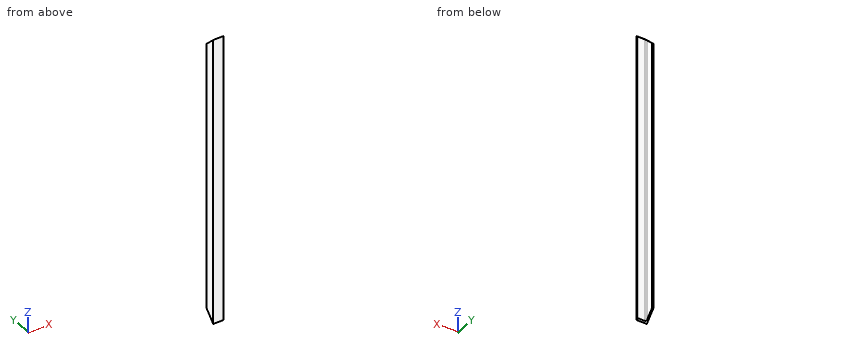
Autodesk Inventor part; units mm, degrees
ref_plane "Start plane" through (0, 0, 0) normal (0, 0, 1) x (1, 0, 0)
ref_plane "End plane" through (0, 0, 1092.2) normal (0, 0, 1) x (1, 0, 0)
ref_plane "Work Plane4" through (19.05, 0, 0) normal (0, 0.7071, -0.7071) x (1, 0, 0)
ref_plane "Start plane" through (0, 0, 0) normal (0, 0, 1) x (1, 0, 0)
ref_plane "End plane" through (0, 0, 1092.2) normal (0, 0, 1) x (1, 0, 0)
sketch "Sketch" plane through (0, 0, 0) normal (0, 0, 1) x (1, 0, 0)
  line L0 (38.1, 0) -> (0, 0)
  line L1 (0, 0) -> (0, 38.1)
  line L2 (0, 38.1) -> (2.4765, 38.1)
  line L3 (4.7625, 35.814) -> (4.7625, 9.5885)
  line L4 (9.5885, 4.7625) -> (35.814, 4.7625)
  line L5 (38.1, 2.4765) -> (38.1, 0)
  line L6 (0, -11.0414) -> (0, 31.5385) construction
  line L7 (-11.0414, 0) -> (31.5385, 0) construction
  arc A0 (4.7625, 9.5885) -> (9.5885, 4.7625) centre (9.5885, 9.5885) ccw
  arc A1 (4.7625, 35.814) -> (2.4765, 38.1) centre (2.4765, 35.814) ccw
  arc A2 (38.1, 2.4765) -> (35.814, 4.7625) centre (35.814, 2.4765) ccw
  line L8 (0, 48.4964) -> (0, -20.9644) construction
  line L9 (-20.9644, 0) -> (48.4964, 0) construction
  point P0 (4.7625, 38.1)
  point P1 (4.7625, 4.7625)
  point P2 (38.1, 4.7625)
  dimension "d0" = 38.1
  dimension "d1" = 38.1
  dimension "d2" = 4.7625
  dimension "d3" = 4.7625
  dimension "d10" = 0
  dimension "d11" = 0
  dimension "d14" = 4.826
  dimension "d15" = 2.286
extrude "Body" add sketch "Sketch" along normal up to surface (1092.2 mm away) from surface at 0
sketch "Sketch3" plane through (0, 0, 0) normal (0, 0, 1) x (1, 0, 0)
  line L0 (0, 0) -> (10, 0)
ref_plane "Work Plane3" through (0, 0, 0) normal (0, -1, 0) x (1, 0, 0)
sketch "Sketch4" plane through (0, 0, 0) normal (0, -1, 0) x (1, 0, 0)
  line L0 (-2, 0) -> (12, 0)
  line L1 (-2, 1092.2) -> (12, 1092.2)
  dimension "d17" = 1092.2
ref_plane "Work Plane4" through (19.05, 0, 0) normal (0, 0.7071, -0.7071) x (1, 0, 0)
split "Split1" plane through (19.05, 0, 0) removes the side toward (0, 0.7071, -0.7071)
ref_plane "Work Plane5" through (19.05, 0, 1092.2) normal (0, 0.7071, 0.7071) x (1, 0, 0)
split "Split2" plane through (19.05, 0, 1092.2) removes the side toward (0, 0.7071, 0.7071)
equation "\"d0\" = G_H"
equation "\"d1\" = G_H"
equation "\"d2\" = G_T"
equation "\"d3\" = G_T"
equation "\"d14\" = G_IR"
equation "\"d15\" = G_ER"
equation "\"d4\" = G_L"
equation "\"G_H\" = 38.1"
equation "\"G_T\" = 4.7625"
equation "\"G_ER\" = 2.286"
equation "\"G_IR\" = 4.826"
equation "\"G_L\" = d17"
equation "\"ex\" = 0"
equation "\"G_OFFSET_START\" = 0"
equation "\"G_OFFSET_END\" = 0"
equation "\"d13\" = G_OFFSET_END + B_L"
equation "\"B_L\" = 1092.2"
properties part number "AISC - L 1.5 x 1.5 x 3/16 - 43" material "Aluminum 6061"
The listing builds one solid part. Answer for the finished solid, in the listing's coordinates (mm). Give positions to 0.01 mm unless a question says otherwise; leave off trailing zeros. Order: outer loops, then holes, each group sorted by start corner. A loop starts at its lowest first (then second) coordinate and runs counter-clockwise, first axis right, second up. Notation, with made-up numbers: (-8.5, 14) - (22.5, 14) arc R22 ccw to (22.5, 41) - close; hole circle Ø5 at (-19.5, -13.5). An arc over 180 degrees is marked (long way). Use one line per item in the form item = value. Start each with the question number.
(1) Flat-ended cylindrical pins translate along their axes: pin 1 Ø8 at (y, z) = (14, 216) entering from +X; pin 2 Ø4 at (x, y) = (23, 4) entering from +Z; pin 3 Ø10 at (y, z) = (11.5, 571.5) entering from +X. Find the tip coordinate at first contact, or state that the pin passes through.
(2) Consider line 1 (X direction, y = 22, z = 981.5); line 2 (Y direction, x = 8.5, z = 665). Determine where each line is inside the solid, lowest interval first. Write a range as from..to.
(3) A cutting plane is placed at B-B, the plane x = 28.5. Write down the section's boundary in (y, z).
(4) A cutting plane is placed at C-C, the plane y = 17. Write down the section's boundary in (x, z), then the cut area to 3 significant figures.
(5) A cutting plane is placed at A-A, the plane z = 582. Write down the section's boundary in (x, y).
Ans:
q1.pin_1 = 4.76
q1.pin_2 = 1090.2
q1.pin_3 = 5.88
q2.line_1 = 0..4.76
q2.line_2 = 0..4.89
q3.outline = (0, 0) - (4.76, 4.76) - (4.76, 1087.44) - (0, 1092.2) - close
q4.outline = (0, 17) - (4.76, 17) - (4.76, 1075.2) - (0, 1075.2) - close
q4.area = 5,040 mm^2
q5.outline = (0, 0) - (38.1, 0) - (38.1, 2.48) arc R2.29 ccw to (35.81, 4.76) - (9.59, 4.76) arc R4.83 cw to (4.76, 9.59) - (4.76, 35.81) arc R2.29 ccw to (2.48, 38.1) - (0, 38.1) - close
